Read the model definition and answer for the solid it produces. Units are mm, in the model's axes. A direction names the side the tool comes from. Give positions to 0.01 mm unless a question says otherwise; leave off trailing zeros. Write each loop counter-clockwise with the first axis right and the second up, starting at its lowest first coordinate (ties: lowest second). Pieces come first, ordered by that corner, then holes. Notation, with made-up numbers: (42, -11) - (58, -11) arc R29 ccw to (58, 11) - close; hole circle Ø3 at (58.25, -22). An arc over 180 degrees is marked (long way). Answer as CSV lines item,"result".
```python
from build123d import *

# Parameters (mm, degrees)
BOSS_EXTRUDE1_DEPTH = 5.7912
FILLET1_R           = 6.35
SKETCH2_R           = 0.1984375
CUT_EXTRUDE1_DEPTH  = 6.7912


with BuildPart() as part:
    # Sketch1 → Boss-Extrude1 (new body)
    with BuildSketch(Plane.XY):
        with BuildLine():
            Line((-6.35, 0), (-9.525, 0))
            Line((-9.525, 0), (-4.7625, -16.1925))
            ThreePointArc((-4.7625, -16.1925), (-3.175, -17.78), (-1.5875, -16.1925))
            Line((-1.5875, -16.1925), (3.175, 0))
            Line((3.175, 0), (0, 0))
            Line((0, 0), (0, 5.7912))
            Line((0, 5.7912), (-6.35, 5.7912))
            Line((-6.35, 5.7912), (-6.35, 0))
        make_face()
    extrude(amount=BOSS_EXTRUDE1_DEPTH)

    # Fillet1
    fillet1_edges = [part.edges().sort_by_distance(p)[0] for p in [
        (-1.5875, -16.1925, 2.8956),
        (-4.7625, -16.1925, 2.8956),
    ]]
    fillet(fillet1_edges, radius=FILLET1_R)

    # Sketch2 → Cut-Extrude1 (cut, through all)
    with BuildSketch(Plane.XY.offset(5.7912)):
        with Locations((-6.35, 0)):
            Circle(SKETCH2_R)
        Circle(SKETCH2_R)
    extrude(amount=-CUT_EXTRUDE1_DEPTH, mode=Mode.SUBTRACT)


solid = part.part
```
(1) A cutting plane is placed at C-C (x = 1.75). Write down the section's boundary in (y, z) (3 decimals).
Worked out:
outline,"(-4.845, 0) - (0, 0) - (0, 5.791) - (-4.845, 5.791) - close"
(2) Each of these flat-tipped pins is pushed along its axis until it touches: P1, Ø1.5, axis at y = 0.5, z = 1, coming from the -X side (3 decimals); P2, Ø0.9, axis at x = -8.5, z = 4, coming from the +Y side; P3, Ø3, axis at y = -2.5, z = 4, coming from the +X side. Where does it stop, or does it pass through?
Worked out:
P1,"stops at x = -9.525"
P2,"stops at y = 0"
P3,"stops at x = 2.88"
(3) For faces 1 (the flat face through (0, 3, 3)), 2 (the flat face through (-3, -6, 5.791)), 3 (the flat face through (-8, 0, 3)), determine the directions among +Z, -Z, +X, -X, +Y, -Y from which every point of the face is accessible in a straight line to the end or side of a thin tool.
Worked out:
face 1,"+Z, -Z, +X, +Y"
face 2,"+Z, +X, -X, +Y, -Y"
face 3,"+Z, -Z, -X, +Y"
(4) Find the intervals of material crossed by L1, parallel to X at y = 0.5, z = 2.05; L2, parallel to Y at x = -3.75, z = 3.6; L3, parallel to X at y = -12.5, z = 1.75, in increasing order.
Worked out:
L1,"x = -6.35 to 0"
L2,"y = -17.67 to 5.79"
L3,"x = -5.85 to -0.5"
(5) A cutting plane is placed at B-B (y = 0.5). Write down the section's boundary in (x, z), and give its area (3 significant figures).
Worked out:
outline,"(-6.35, 0) - (0, 0) - (0, 5.79) - (-6.35, 5.79) - close"
area,"36.8 mm^2"
